Source: CAD feature listing. Evaluate the final solid. Frame: model axes, mm. A direction names the side the tool comes from. Give positions to 0.01 mm unless a question says otherwise; leave off trailing zeros. Loops run counter-clockwise (first coordinate to the right, second up) from the corner with the lowest first, then second, coordinate; pieces in that order, holes last. Notation, with made-up numbers: M 24.5,87.5 L 43.5,87.5 A17 ccw 43.5,97.5 Z; hole C 55,13 d11. An arc over 180 degrees is marked long. Answer in a Markdown table with one row per item.
```python
from build123d import *

# Parameters (mm, degrees)
SKETCH2_W           = 54
SKETCH2_H           = 50
SKETCH2_R           = 5
SKETCH2_R_2         = 2
BOSS_EXTRUDE1_DEPTH = 5
SKETCH3_W           = 14
SKETCH3_H           = 5
SKETCH3_W_2         = 10
SKETCH3_W_3         = 54
BOSS_EXTRUDE2_DEPTH = 21
SKETCH3_3_W         = 74
SKETCH3_3_H         = 5
BOSS_EXTRUDE3_DEPTH = 5
SKETCH3_4_W         = 10
SKETCH3_4_H         = 5
BOSS_EXTRUDE4_DEPTH = 5
SKETCH4_R           = 13.25
CUT_EXTRUDE1_DEPTH  = 2.5
BOSS_EXTRUDE7_DEPTH = 4
BOSS_EXTRUDE8_START = -50
BOSS_EXTRUDE8_DEPTH = 4


with BuildPart() as part:
    # Sketch2 → Boss-Extrude1 (new body)
    with BuildSketch(Plane.XY):
        Rectangle(SKETCH2_W, SKETCH2_H)
        Circle(SKETCH2_R, mode=Mode.SUBTRACT)
        with Locations((-12.840811795, 11.889640551)):
            Circle(SKETCH2_R_2, mode=Mode.SUBTRACT)
        with Locations(Location((-12.840811795, -11.889640551, 0), (0, 0, 180))):
            Circle(SKETCH2_R_2, mode=Mode.SUBTRACT)
        with Locations((12.840811795, -11.889640551)):
            Circle(SKETCH2_R_2, mode=Mode.SUBTRACT)
        with Locations(Location((12.840811795, 11.889640551, 0), (0, 0, 180))):
            Circle(SKETCH2_R_2, mode=Mode.SUBTRACT)
    extrude(amount=BOSS_EXTRUDE1_DEPTH)

    # Sketch3 → Boss-Extrude2 (add)
    with BuildSketch(Plane.XY.offset(5)):
        with Locations((-20, -22.5)):
            Rectangle(SKETCH3_W, SKETCH3_H)
        with Locations((-32, -22.5)):
            Rectangle(SKETCH3_W_2, SKETCH3_H)
        with Locations((20, -22.5)):
            Rectangle(SKETCH3_W, SKETCH3_H)
        with Locations((32, -22.5)):
            Rectangle(SKETCH3_W_2, SKETCH3_H)
        with Locations((0, 22.5)):
            Rectangle(SKETCH3_W_3, SKETCH3_H)
        with Locations((-32, 22.5)):
            Rectangle(SKETCH3_W_2, SKETCH3_H)
        with Locations((32, 22.5)):
            Rectangle(SKETCH3_W_2, SKETCH3_H)
    extrude(amount=BOSS_EXTRUDE2_DEPTH)

    # Sketch3_3 → Boss-Extrude3 (add)
    with BuildSketch(Plane.XY.offset(5)):
        with Locations((0, 22.5)):
            Rectangle(SKETCH3_3_W, SKETCH3_3_H)
    extrude(amount=-BOSS_EXTRUDE3_DEPTH)

    # Sketch3_4 → Boss-Extrude4 (add)
    with BuildSketch(Plane.XY.offset(5)):
        with Locations((32, -22.5)):
            Rectangle(SKETCH3_4_W, SKETCH3_4_H)
        with Locations((-32, -22.5)):
            Rectangle(SKETCH3_4_W, SKETCH3_4_H)
    extrude(amount=-BOSS_EXTRUDE4_DEPTH)

    # Sketch4 → Cut-Extrude1 (cut)
    with BuildSketch(Plane.XY.offset(5)):
        Circle(SKETCH4_R)
    extrude(amount=-CUT_EXTRUDE1_DEPTH, mode=Mode.SUBTRACT)

    # Sketch5 → Boss-Extrude7 (add)
    with BuildSketch(Plane(origin=(27, 0, 0), x_dir=(0, 0, -1), z_dir=(1, 0, 0))):
        Polygon((-26, 20), (-5, 2.126814834), (-5, 20), align=None)
        Polygon((-26, -20), (-5, -20), (-5, -2.126814834), align=None)
    extrude(amount=-BOSS_EXTRUDE7_DEPTH)

    # Sketch5_2 → Boss-Extrude8 (add)
    with BuildSketch(Plane(origin=(27, 0, 0), x_dir=(0, 0, -1), z_dir=(1, 0, 0)).offset(BOSS_EXTRUDE8_START)):
        Polygon((-26, 20), (-5, 2.126814834), (-5, 20), align=None)
        Polygon((-26, -20), (-5, -20), (-5, -2.126814834), align=None)
    extrude(amount=-BOSS_EXTRUDE8_DEPTH)


solid = part.part
```
Q1. Section query D-D (x = -20.5). Output: boundary loops of the cut face in (y, z), plus the area to 3 significant figures.
Values follow:
| item | result |
|---|---|
| outline | M -25,0 L 25,0 L 25,26 L 20,26 L 20,5 L -20,5 L -20,26 L -25,26 Z |
| area | 460 mm^2 |
Q2. Mould query, pull axis X, two halves, no side actions, for faces 1 (the flat face through (-0.5, -25, 4.5)), 2 (the flat face through (-18, -20, 15)), 3 (the flat face through (37, -23, 13)), 4 (the flat face through (-13, -23, 15)). Classes: +X half, -X half, draft (parallel to the pull), parting line (faces both ways), or undercut.
Values follow:
| item | result |
|---|---|
| face 1 | draft |
| face 2 | undercut |
| face 3 | +X half |
| face 4 | undercut |
Q3. Section query A-A (x = 0). Output: boundary loops of the cut face in (y, z), plus the area to 3 significant figures.
Values follow:
| item | result |
|---|---|
| outline | M -25,0 L -5,0 L -5,2.5 L -13.25,2.5 L -13.25,5 L -25,5 Z; M 5,0 L 25,0 L 25,26 L 20,26 L 20,5 L 13.25,5 L 13.25,2.5 L 5,2.5 Z |
| area | 264 mm^2 |
Q4. Contact query for flat-ended pins moving along their axis: pin 1 Ø13 at (y, z) = (-5.5, 12.5) entering from +X; pin 2 Ø14.5 at (y, z) = (11, 14) entering from -X; pin 3 Ø8 at (x, y) = (-15.5, 9.5) entering from +Z. Output: stop coordinate, or through.
Values follow:
| item | result |
|---|---|
| pin 1 | x = 27 |
| pin 2 | x = -27 |
| pin 3 | z = 5 |
Q5. Section query C-C (z = 21). Output: boundary loops of the cut face in (x, y), plus the area to 3 significant figures.
Values follow:
| item | result |
|---|---|
| outline | M -37,-25 L -13,-25 L -13,-20 L -23,-20 L -23,-15.74 L -27,-15.74 L -27,-20 L -37,-20 Z; M -37,20 L -27,20 L -27,15.74 L -23,15.74 L -23,20 L 23,20 L 23,15.74 L 27,15.74 L 27,20 L 37,20 L 37,25 L -37,25 Z; M 13,-25 L 37,-25 L 37,-20 L 27,-20 L 27,-15.74 L 23,-15.74 L 23,-20 L 13,-20 Z |
| area | 678 mm^2 |
Q6. Section query B-B (y = 0). Output: boundary loops of the cut face in (x, z).
Values follow:
| item | result |
|---|---|
| outline | M -27,0 L -5,0 L -5,2.5 L -13.25,2.5 L -13.25,5 L -27,5 Z; M 5,0 L 27,0 L 27,5 L 13.25,5 L 13.25,2.5 L 5,2.5 Z |
Q7. Ray query, probe 1 along X at (y, z) = (-14.5, 15.75); probe 2 along Y at (x, z) = (21, 11.25); probe 3 along Y at (x, z) = (0, 1.1). Return the intervals inside material, ascending. Write a range as from..to.
Values follow:
| item | result |
|---|---|
| probe 1 | -27..-23, 23..27 |
| probe 2 | -25..-20, 20..25 |
| probe 3 | -25..-5, 5..25 |
Q8. Reachability of faces 5 (the flat face through (25.028, -10.938, 15.353)), 6 (the flat face through (-1, 23, 26)), 7 (the flat face through (23, 15, 11)), 8 (the flat face through (32, 20, 13)) from +Z, -Z, +X, -X, +Y, -Y: full face, straight path, thin tool, end or side. Return the list, or none.
Values follow:
| item | result |
|---|---|
| face 5 | +Z, +X, -X |
| face 6 | +Z, +X, -X, +Y, -Y |
| face 7 | +Z |
| face 8 | +Z, -Z, +X |
